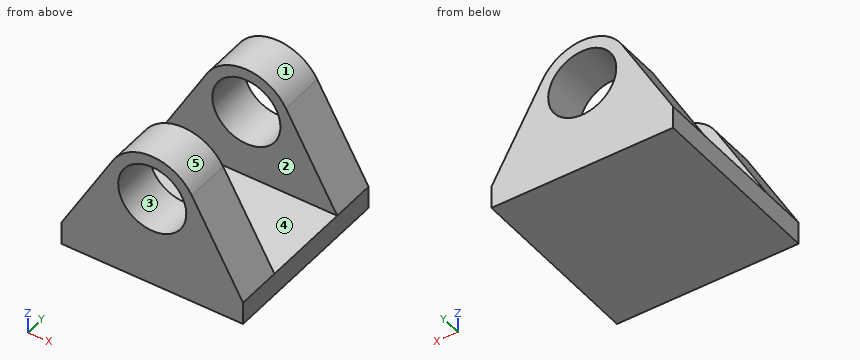
```python
from build123d import *

# Parameters (mm, degrees)
SKETCH_2_W          = 80
SKETCH_2_H          = 80
EXTRUDE_1_DEPTH     = 10
EXTRUDE_2_DEPTH     = 20
EXTRUDE_START       = -20
EXTRUDE_3_DEPTH     = 20
SKETCH_5_R          = 15
CUT_EXTRUDE_1_DEPTH = 80


with BuildPart() as part:
    # 草图2 → 凸台-拉伸1 (new body)
    with BuildSketch(Plane.XY):
        with Locations((40, 40)):
            Rectangle(SKETCH_2_W, SKETCH_2_H)
    extrude(amount=EXTRUDE_1_DEPTH)

    # 草图3 → 凸台-拉伸2 (add)
    with BuildSketch(Plane.XZ):
        with BuildLine():
            Line((0, 10), (22.601818332, 49.864242224))
            ThreePointArc((22.601818332, 49.864242224), (40, 60), (57.398181668, 49.864242224))
            Line((57.398181668, 49.864242224), (80, 10))
            Line((80, 10), (0, 10))
        make_face()
    extrude(amount=-EXTRUDE_2_DEPTH)

    # 草图4 → 凸台-拉伸3 (add)
    with BuildSketch(Plane(origin=(0, 80, 0), x_dir=(1, 0, 0), z_dir=(0, 1, 0)).offset(EXTRUDE_START)):
        with BuildLine():
            Line((80, -10), (57.398181668, -49.864242224))
            ThreePointArc((57.398181668, -49.864242224), (40, -60), (22.601818332, -49.864242224))
            Line((22.601818332, -49.864242224), (0, -10))
            Line((0, -10), (80, -10))
        make_face()
    extrude(amount=EXTRUDE_3_DEPTH)

    # 草图5 → 切除-拉伸1 (cut)
    with BuildSketch(Plane(origin=(0, 80, 0), x_dir=(1, 0, 0), z_dir=(0, 1, 0))):
        with Locations(Location((40, -40, 0), (0, 0, 270))):
            Circle(SKETCH_5_R)
    extrude(amount=-CUT_EXTRUDE_1_DEPTH, mode=Mode.SUBTRACT)


solid = part.part
```
The listing builds one solid part. Answer for the finished solid, in the listing's coordinates (mm). Face numbers are marked on the shaded views. A direction names the side the tool comes from. Give positions to 0.01 mm unless a question says otherwise; leave off trailing zeros. Write each loop counter-clockwise with the first axis right and the second up, starting at its lowest first coordinate (ties: lowest second). Pieces come first, ordered by that corner, then holes. Notation, with made-up numbers: (46.25, -16.5) -> (102.25, -16.5) arc R23 cw to (102.25, 18.5) -> close; hole circle Ø6 at (25, 10.5). An arc over 180 degrees is marked (long way). Write item = value, one per line. Start each with the question number.
1) Straight lines are drawn through the part: line 1 along Y through (x, z) = (63, 26.5); line 2 along Z through (x, y) = (50.5, 38.5); line 3 along X through (y, z) = (74, 40). For each, find the intervals that lie inside material, in ascending order.
2) The part is cut by section B-B, the plane z = 40. Determine the outline of the cut face in (x, y).
3) The part is cut by section D-D, the plane z = 22.5. Determine the outline of the cut face in (x, y).
4) Each of these flat-tipped pins is pushed along its axis until it touches: pin 1 (8 mm diameter, centred on x = 25, y = 26, fed in from +Z); pin 2 (4 mm diameter, centred on y = 68.5, z = 49.5, fed in from +X); pin 3 (24 mm diameter, centred on x = 40, z = 40, fed in from +Y); pin 4 (2 mm diameter, centred on x = 52.5, y = 14.5, fed in from +Z). Where does it stop, or does it pass through?
5) Determine the mould class of the marked faces 1, 2 and 3 for opening direction Z: +Z half, -Z half, draft (parallel to the pull), parting line (faces both ways), or undercut.
6) Which of the six approach directions +Z, -Z, +X, -X, +Y, -Y give full straight-line access (tool end or side, diameter ignored) to the marked faces 4 and 5?
7) The part is cut by section A-A, the plane x = 40. Determine the outline of the cut face in (y, z).
8) The part is cut by section C-C, the plane y = 68. Determine the outline of the cut face in (x, z), and give its area (3 significant figures).
Solutions:
q1.line_1 = 0 to 20, 60 to 80
q1.line_2 = 0 to 10
q1.line_3 = 17.01 to 25, 55 to 62.99
q2.outline = (17.01, 0) -> (25, 0) -> (25, 20) -> (17.01, 20) -> close; (17.01, 60) -> (25, 60) -> (25, 80) -> (17.01, 80) -> close; (55, 0) -> (62.99, 0) -> (62.99, 20) -> (55, 20) -> close; (55, 60) -> (62.99, 60) -> (62.99, 80) -> (55, 80) -> close
q3.outline = (7.09, 0) -> (72.91, 0) -> (72.91, 20) -> (7.09, 20) -> close; (7.09, 60) -> (72.91, 60) -> (72.91, 80) -> (7.09, 80) -> close
q4.pin_1 = 10
q4.pin_2 = 58.74
q4.pin_3 = through
q4.pin_4 = 56.36
q5.face_1 = +Z half
q5.face_2 = draft
q5.face_3 = undercut
q6.face_4 = +Z, +X, -X
q6.face_5 = +Z, +Y, -Y
q7.outline = (0, 0) -> (80, 0) -> (80, 25) -> (60, 25) -> (60, 10) -> (20, 10) -> (20, 25) -> (0, 25) -> close; (0, 55) -> (20, 55) -> (20, 60) -> (0, 60) -> close; (60, 55) -> (80, 55) -> (80, 60) -> (60, 60) -> close
q8.outline = (0, 0) -> (80, 0) -> (80, 10) -> (57.4, 49.86) arc R20 ccw to (22.6, 49.86) -> (0, 10) -> close; hole circle Ø30 at (40, 40)
q8.area = 2,630 mm²
